Autodesk Inventor part; units mm, degrees
ref_plane "YZ Plane" through (0, 0, 0) normal (1, 0, 0) x (0, 1, 0)
ref_plane "XZ Plane" through (0, 0, 0) normal (0, 1, 0) x (-1, 0, 0)
ref_plane "XY Plane" through (0, 0, 0) normal (0, 0, 1) x (1, 0, 0)
sketch "Sketch1" plane through (0, 0, 0) normal (0, 0, 1) x (1, 0, 0)
  circle A0 centre (0, 0) radius 35
  circle A1 centre (270, -72) radius 35
  line L0 (0, 35) -> (212.4975, 35)
  line L1 (212.4975, 35) -> (294.7487, -47.2513)
  line L2 (0, -35) -> (183.5025, -35)
  line L3 (183.5025, -35) -> (245.2513, -96.7487)
  dimension "d0" = 70
  dimension "d1" = 70
  dimension "d2" = 135
  dimension "d3" = 37
  dimension "d4" = 270
extrude "Extrusion1" add sketch "Sketch1" along normal blind 22.5
sketch "Sketch2" plane through (0, 0, 22.5) normal (0, 0, 1) x (1, 0, 0)
  circle A0 centre (0, 0) radius 2.5
  line L0 (-18, 10) -> (29, 10)
  line L1 (29, 10) -> (29, -10)
  line L2 (29, -10) -> (-18, -10)
  line L3 (-18, -10) -> (-18, 10)
  line L4 (-11, 10) -> (36, 10)
  line L5 (36, 10) -> (36, -10)
  line L6 (36, -10) -> (-11, -10)
  line L7 (-11, -10) -> (-11, 10)
  line L8 (-18, 0) -> (36, 0) construction
  point P0 (29, 10)
  dimension "d7" = 5
  dimension "d9" = 54
  dimension "d10" = 40
  dimension "d11" = 7
  dimension "d12" = 36
  dimension "d13" = 20
extrude "Extrusion2" cut sketch "Sketch2" against normal through all contours A0 | L0 L1 L2 L7
extrude "Extrusion3" cut sketch "Sketch2" against normal blind 13.5 contours L0 L7 L2 L3 | L4 L5 L6 L1
sketch "Sketch3" plane through (0, 0, 0) normal (0, 0, -1) x (-1, 0, 0)
  arc A0 (-294.7487, -47.2513) -> (-245.2513, -96.7487) centre (-270, -72) ccw
  line L0 (-183.5025, -35) -> (-245.2513, -96.7487)
  line L1 (0, -35) -> (-183.5025, -35)
  arc A1 (0, -35) -> (0, 35) centre (0, 0) ccw
  line L2 (-212.4975, 35) -> (0, 35)
  line L3 (-294.7487, -47.2513) -> (-212.4975, 35)
  line L4 (0, -35) -> (-183.5025, -35)
  line L5 (-212.4975, 35) -> (-142.4975, -35)
  point P0 (-142.4975, -35)
  dimension "d18" = 135
extrude "Extrusion4" add sketch "Sketch3" along normal blind 12.5 contours L3 L5 L1 L0 A0
chamfer "Chamfer1" distance 12.5 angle 45 1 edges at (177.4975, 0, 0)
sketch "Sketch4" plane through (0, 0, 22.5) normal (0, 0, 1) x (1, 0, 0)
  line L0 (183.5025, -35) -> (245.2513, -96.7487)
  arc A0 (245.2513, -96.7487) -> (294.7487, -47.2513) centre (270, -72) ccw
  line L1 (294.7487, -47.2513) -> (212.4975, 35)
  line L2 (212.4975, 35) -> (0, 35)
  arc A1 (0, 35) -> (0, -35) centre (0, 0) ccw
  line L3 (0, -35) -> (183.5025, -35)
  line L4 (183.5025, -35) -> (245.2513, -96.7487)
  line L5 (-18, 10) -> (36, 10)
  line L6 (36, 10) -> (36, -10)
  line L7 (36, -10) -> (-18, -10)
  line L8 (-18, -10) -> (-18, 10)
  line L9 (245.2513, -96.7487) -> (183.5025, -35)
  line L10 (183.5025, -35) -> (282.4975, -35)
extrude "Extrusion5" cut sketch "Sketch4" against normal blind 22.5 contours L10 L1 A0 L0
sketch "Sketch5" plane through (0, 0, 0) normal (0, 0, 1) x (1, 0, 0)
  arc A0 (245.2513, -96.7487) -> (294.7487, -47.2513) centre (270, -72) ccw
  circle A1 centre (270, -72) radius 12.5
  point P0 (0, 0)
  dimension "d26" = 25
extrude "Extrusion6" cut sketch "Sketch5" against normal blind 7
properties part number "arm 1 right"
Verification items for the finished model (mm, model axes). A direction names the side the tool comes from. Coordinates: 2 decimals unless noted, no trailing zeros. Write each loop counter-clockwise with the first axis right and the second up, starting at its lowest first coordinate (ties: lowest second). Pieces come first, ordered by that corner, then holes. Notation, with made-up numbers: (49.25, 63.5) -> (82.25, 63.5) arc R21 ccw to (82.25, 81.5) -> close; hole circle Ø8 at (10, -12). An arc over 180 degrees is marked (long way). One line per item, written item: value. Start each with the question number.
Q1. Mould release check, pull along X, two halves, no side actions. Record for faces 1 (the flat face through (29, 0, 5)), 2 (the flat face through (78, 0, 0)), 3 (the flat face through (169.149, 0.614, -6.162)): pulls with the +X half, pulls with the -X half, needs draft (parallel to the pull), parting line crosses it, or undercut.
Q2. Cross-section at C-C on x = 270. Enter the section's corners in (y, z), and give its area (3 significant figures).
Q3. Access from +Z, -Z, +X, -X, +Y, -Y to the whole of each face (thin tool, end or side, straight path). Record for faces 4 (the cylindrical face through (281.923, -68.245, -3.451)), 5 (the flat face through (254.2, -6.7, 5.2)), 6 (the flat face through (257, -62, 0)), 7 (the flat face through (-11, 0, 5)), 8 (the cylindrical face through (-34.99, -0.77, 11.09)).
Q4. Thickness scan on L1, parallel to Y at x = 33, z = 14; L2, parallel to Y at x = 270, z = -4; L3, parallel to Y at x = 190.5, z = 8. Record the ranges inside material, lowest first. Write a range as from..to.
Q5. Cross-section at A-A on z = 16.5. Enter the section's corners in (x, y), and give its area (3 significant figures).
Q6. Go/stop test with flat-tipped pins: P1, Ø4, axis at x = 132, y = -8, coming from the -Z side; P2, Ø3, axis at y = -26, z = 15, coming from the +X side; P3, Ø1.5, axis at x = 28, y = -6.5, coming from the +Z side; P4, Ø17.5, axis at x = 81.5, z = 6.5, coming from the -Y side. Record where each tip stops, or that it passes through.
Checked values:
1. face 1: undercut
1. face 2: needs draft
1. face 3: pulls with the -X half
2. outline: (-107, -12.5) -> (-22.5, -12.5) -> (-22.5, 22.5) -> (-35, 22.5) -> (-35, 0) -> (-59.5, 0) -> (-59.5, -7) -> (-84.5, -7) -> (-84.5, 0) -> (-107, 0) -> close
2. area: 1,160 mm²
3. face 4: +Z
3. face 5: +Z, -Z, +X, +Y
3. face 6: +Z, +X, -X, -Y
3. face 7: +Z, -Z
3. face 8: +Z, -Z, -X
4. L1: y = -35..-10, 10..35
4. L2: y = -107..-84.5, -59.5..-22.5
4. L3: y = -35..35
5. outline: (0, -35) -> (282.5, -35) -> (212.5, 35) -> (0, 35) arc R35 ccw to start; hole (-18, -10) -> (36, -10) -> (36, 10) -> (-18, 10) -> close
5. area: 18,200 mm²
6. P1: stops at z = 0
6. P2: stops at x = 275
6. P3: passes through
6. P4: stops at y = -35
